Source: three-view drawing plus pictorial views. Frame: mm from the lowest corner of the part. A direction names the side the tool comes from. Give positions to 0.01 mm unless a question says otherwise; leave off trailing zeros. Order: outer loops, then holes, each group sorted by start corner. A loop starts at its lowest first (then second) coordinate and runs counter-clockwise, first axis right, second up.
1) Section B-B, the plane x = 7.05. Return loops of the section in (y, z), plus the area to 3 significant figures.
2) Material intervals for line 1 (Z direction, x = 7.05, y = 6.2); line 2 (Y direction, x = 4.5, z = 18.25); line 3 (X direction, y = 7.9, z = 4.5), sorted ascending.
3) Section D-D, the plane x = 4.75. Return loops of the section in (y, z).
4) First-contact query: P1, Ø2.5, axis at y = 7.5, z = 4.5, coming from the +X side; P2, Ø1.5, axis at x = 4.5, z = 4.5, coming from the -Y side; P3, Ø3, axis at y = 2.5, z = 7, coming from the +X side; P4, Ø2.5, axis at y = 6.5, z = 7, coming from the -X side. Flat tips, straight axial feed; report the tip coordinate or a pass-through.
5) Section C-C, the plane y = 6.5. Return loops of the section in (x, z).
6) Section A-A, the plane z = 4.5. Return loops of the section in (x, y).
7) Access query for the marked faces 5, 6, 7, 8 and 9. Directions: +Z, -Z, +X, -X, +Y, -Y. A direction counts if a zero-diameter tool reaches every point of the face in a straight line with its end or side. Return the directions, or none.
8) Draft query along X for the marked faces 1, 2, 3 and 4. Return one class per face: released by +X, released by -X, zero draft, split by the parting line, or undercut.
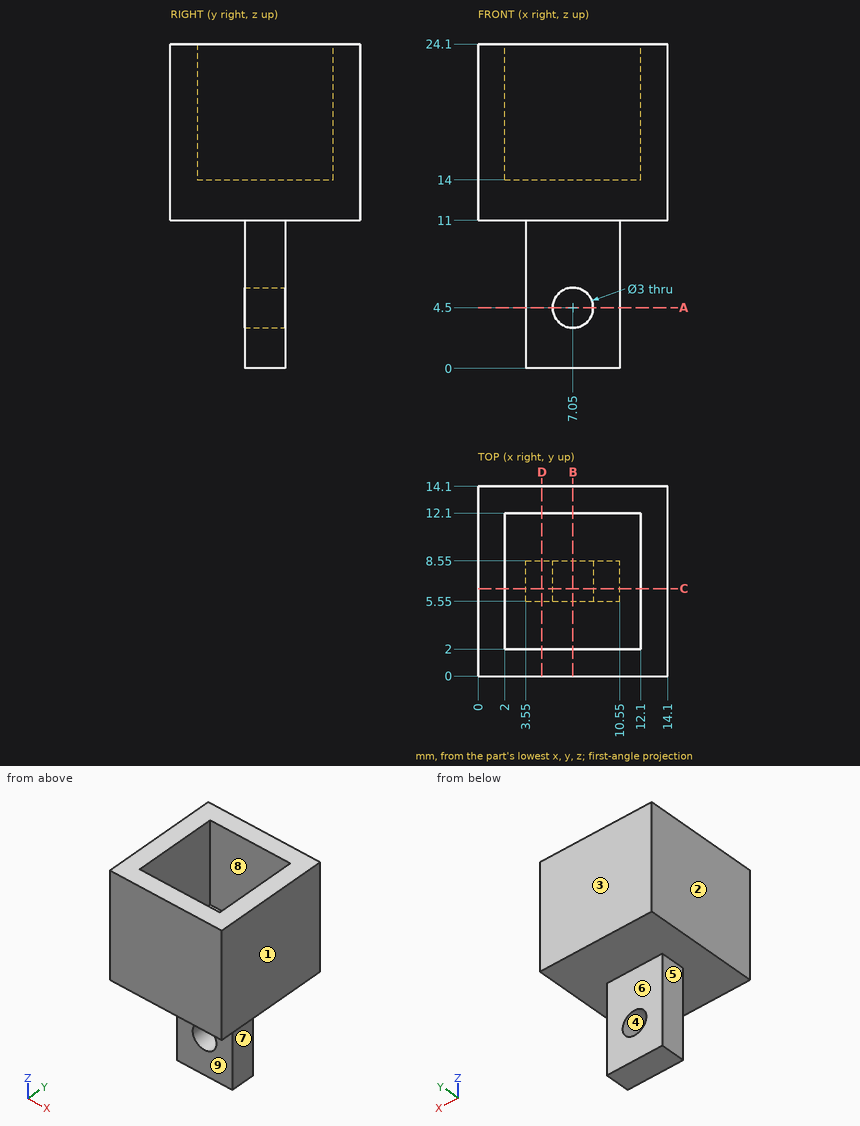
From the geometry:
1. outline: (0, 11) - (5.55, 11) - (5.55, 6) - (8.55, 6) - (8.55, 11) - (14.1, 11) - (14.1, 24.1) - (12.1, 24.1) - (12.1, 14) - (2, 14) - (2, 24.1) - (0, 24.1) - close; (5.55, 0) - (8.55, 0) - (8.55, 3) - (5.55, 3) - close
1. area: 107 mm2
2. line 1: z = 0 to 3, 6 to 14
2. line 2: y = 0 to 2, 12.1 to 14.1
2. line 3: x = 3.55 to 5.55, 8.55 to 10.55
3. outline: (0, 11) - (5.55, 11) - (5.55, 0) - (8.55, 0) - (8.55, 11) - (14.1, 11) - (14.1, 24.1) - (12.1, 24.1) - (12.1, 14) - (2, 14) - (2, 24.1) - (0, 24.1) - close
4. P1: stops at x = 10.55
4. P2: stops at y = 5.55
4. P3: passes through
4. P4: stops at x = 3.55
5. outline: (0, 11) - (3.55, 11) - (3.55, 0) - (10.55, 0) - (10.55, 11) - (14.1, 11) - (14.1, 24.1) - (12.1, 24.1) - (12.1, 14) - (2, 14) - (2, 24.1) - (0, 24.1) - close; hole circle Ø3 at (7.05, 4.5)
6. outline: (3.55, 5.55) - (5.55, 5.55) - (5.55, 8.55) - (3.55, 8.55) - close; (8.55, 5.55) - (10.55, 5.55) - (10.55, 8.55) - (8.55, 8.55) - close
7. face 5: -Z, -X, +Y, -Y
7. face 6: -Z, +X, -X, +Y
7. face 7: -Z, +X, +Y, -Y
7. face 8: +Z
7. face 9: -Z, +X, -X, -Y
8. face 1: released by +X
8. face 2: released by -X
8. face 3: zero draft
8. face 4: undercut
